Build history of the part. All positions in model axes, mm. Round coordinates to 2 decimals unless told otherwise and drop trailing zeros. Order: outer loops, then holes, each group sorted by start corner. A loop starts at its lowest first (then second) coordinate and runs counter-clockwise, first axis right, second up. Notation, with made-up numbers: (-19.5, -1.75) -> (36.5, -1.75) arc R33 ccw to (36.5, 32.25) -> close; hole circle Ø11 at (27.25, 34.25). An arc over 180 degrees is marked (long way). Answer as a JSON object with one key per item and string values.
Autodesk Fusion 360 part; units mm, degrees
sketch "Esboço1" plane through (0, 0, 0) normal (0, 1, 0) x (1, 0, 0)
  line L0 (0, 7.9375) -> (0, 93.6625)
  line L1 (15.875, 93.6625) -> (15.875, 7.9375)
  arc A0 (0, 7.9375) -> (15.875, 7.9375) centre (7.9375, 7.9375) ccw
  arc A1 (15.875, 93.6625) -> (0, 93.6625) centre (7.9375, 93.6625) ccw
  line L2 (7.9375, 38.1) -> (7.9375, 38)
  line L3 (7.9375, 6.35) -> (7.9375, 7.9375)
  circle A2 centre (7.9375, 6.35) radius 2.108
  circle A3 centre (7.9375, 12.7) radius 2.108
  circle A4 centre (7.9375, 19.05) radius 2.108
  circle A5 centre (7.9375, 25.4) radius 2.108
  circle A6 centre (7.9375, 31.75) radius 2.108
  circle A7 centre (7.9375, 38.1) radius 2.108
  line L4 (7.9375, 12.7) -> (7.9375, 14.808)
  arc A8 (10.4775, 94.767) -> (5.3975, 94.767) centre (7.9375, 94.767) ccw
  arc A9 (5.3975, 44.704) -> (10.4775, 44.704) centre (7.9375, 44.704) ccw
  line L5 (5.3975, 94.767) -> (5.3975, 44.704)
  line L6 (10.4775, 94.767) -> (10.4775, 44.704)
  dimension "d7" = 6.35
  dimension "d8" = 6.35
  dimension "d9" = 6.35
  dimension "d10" = 6.35
  dimension "d11" = 6.35
  dimension "d12" = 4.216
  dimension "d13" = 4.216
  dimension "d14" = 4.216
  dimension "d15" = 4.216
  dimension "d16" = 4.216
  dimension "d17" = 4.216
  dimension "d19" = 5.08
  dimension "d20" = 50.063
  dimension "d21" = 5.08
extrude "Extrusão1" add sketch "Esboço1" along normal blind 4.699
chamfer "Chanfro1" distance 0.3 angle 45 14 edges at (15.875, 4.699, -50.8) (7.9375, 4.699, -101.6) (0, 4.699, -50.8) (7.9375, 4.699, 0) (10.4775, 4.699, -69.7355) (7.9375, 4.699, -42.164) (5.3975, 4.699, -69.7355) (7.9375, 4.699, -97.307) (5.9722, 4.699, -38.8623) (5.9722, 4.699, -32.5123) (5.9722, 4.699, -26.1623) (5.9722, 4.699, -19.8123) (5.9722, 4.699, -13.4623) (5.9722, 4.699, -7.1123)
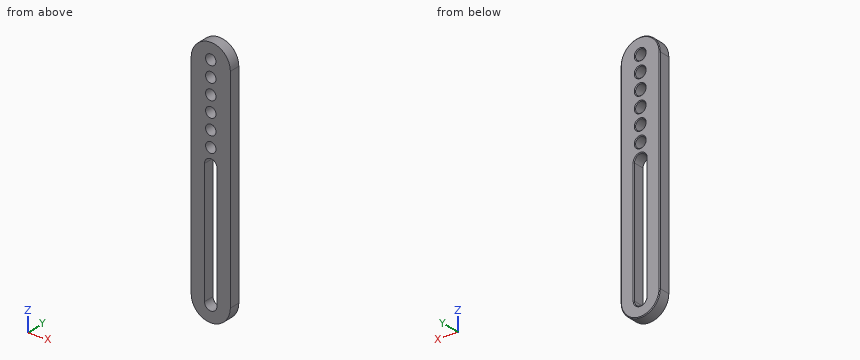
1) Cut at A-A, the plane z = -38.1. Give the cut face in (x, y) (1 decimal).
Checked values:
{"outline": "(0, 0) -> (5.8, 0) -> (5.8, 4.4) -> (5.5, 4.7) -> (0.3, 4.7) -> (0, 4.4) -> close; (10, 0) -> (15.9, 0) -> (15.9, 4.4) -> (15.6, 4.7) -> (10.3, 4.7) -> (10, 4.4) -> close"}
2) Probe L1, parallel to X at y = 3.15, z = -12.7 (1 decimal); L2, parallel to X at y = 2.2, z = -73.5 (1 decimal); L3, parallel to Z at x = 12.5, y = 1.45. List the from-to ranges inside material, lowest first. Write a range as from..to.
Checked values:
{"L1": "x = 0..5.8, 10..15.9", "L2": "x = 0..5.4, 10.5..15.9", "L3": "z = -100.16..-1.44"}
3) Cut at C-C, the plane z = -83. Give the cut face in (x, y) (1 decimal).
Checked values:
{"outline": "(0, 0) -> (5.4, 0) -> (5.4, 4.4) -> (5.1, 4.7) -> (0.3, 4.7) -> (0, 4.4) -> close; (10.5, 0) -> (15.9, 0) -> (15.9, 4.4) -> (15.6, 4.7) -> (10.8, 4.7) -> (10.5, 4.4) -> close"}
4) Cut at B-B, the plane y = 1.3. Count the separate pieces of the cut face and the enclosed holes in it, plus the area to 3 significant figures.
Checked values:
{"separate pieces": "1", "enclosed holes": "7", "area": "1,200 mm²"}
